The drawing under review shows one solid part. Ordinate dimensions are in mm from its lowest x, y, z. A direction names the side the tool comes from. Round coordinates to 2 decimals unless told otherwise and drop trailing zeros. Order: outer loops, then holes, each group sorted by start corner. A loop starts at its lowest first (then second) coordinate and runs counter-clockwise, first axis right, second up. Notation, with made-up numbers: (-8.75, 79) - (31.25, 79) arc R9 ccw to (31.25, 95) - close; hole circle Ø7 at (68, 47). An arc over 180 degrees is marked (long way). One line per question, with ' | ' between items.
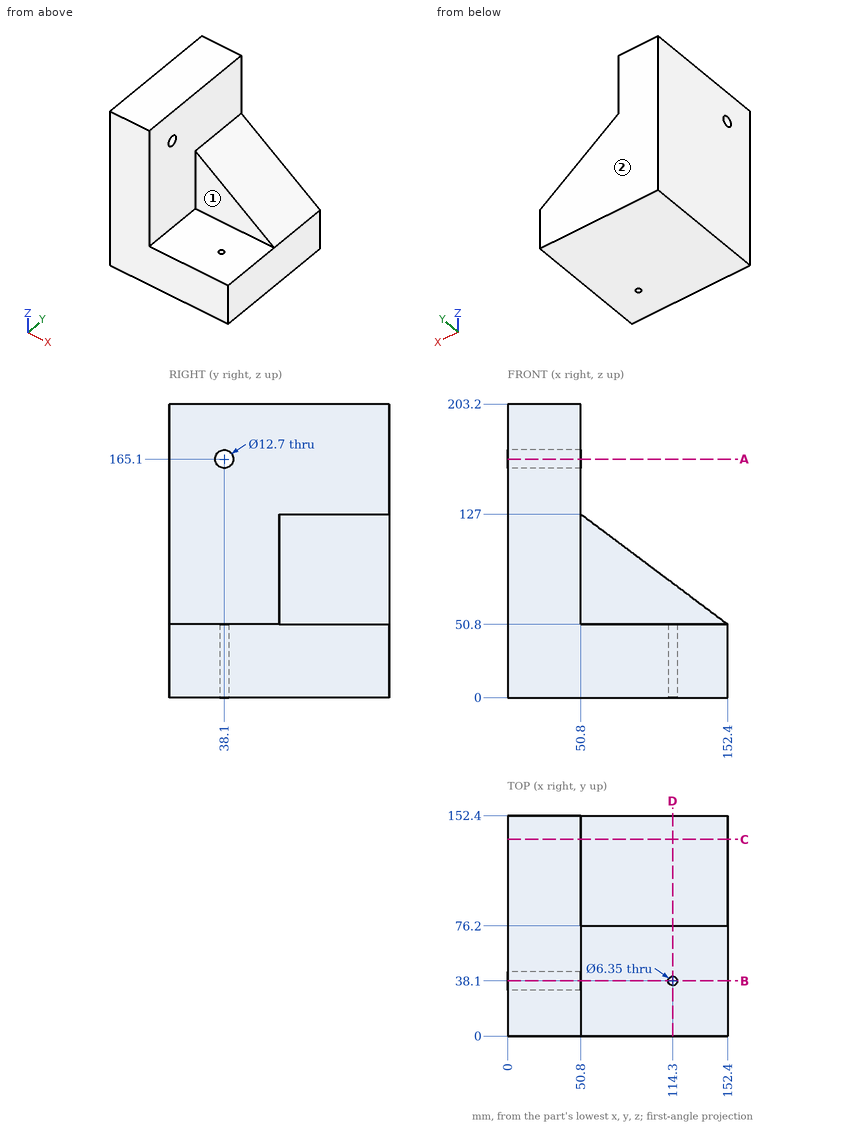
(1) We need section B-B on y = 38.1. State the section outline as (x, z) points (3 decimals), plus the area to 3 significant figures.
Output values:
outline: (0, 0) - (111.125, 0) - (111.125, 50.8) - (50.8, 50.8) - (50.8, 158.75) - (0, 158.75) - close; (0, 171.45) - (50.8, 171.45) - (50.8, 203.2) - (0, 203.2) - close; (117.475, 0) - (152.4, 0) - (152.4, 50.8) - (117.475, 50.8) - close | area: 14,500 mm^2
(2) For the marked faces 1 and 2, list the 3-axis set-ups (+Z, -Z, +X, -X, +Y, -Y) from which the entire face can be reached by the end or side of a thin tool; tool diameter is ignored.
Output values:
face 1: +Z, +X, -Y | face 2: +Z, -Z, +X, -X, +Y
(3) We need section D-D on x = 114.3. State the section outline as (y, z) points (3 decimals), plus the area to 3 significant figures.
Output values:
outline: (0, 0) - (34.925, 0) - (34.925, 50.8) - (0, 50.8) - close; (41.275, 0) - (152.4, 0) - (152.4, 79.375) - (76.2, 79.375) - (76.2, 50.8) - (41.275, 50.8) - close | area: 9,600 mm^2
(4) Insertion check: pin 1 (10 mm diameter, centred on x = 133, y = 99, fed in from +Z); pin 2 (23 mm diameter, centred on x = 124.5, y = 46, fed in from +Z); pin 3 (12 mm diameter, centred on x = 131, y = 106.5, fed in from +Z); pin 4 (6 mm diameter, centred on y = 100.5, z = 52, fed in from +X). Each pin has a flat end and moves straight along its axis. Give the tip position at first contact, or say it passes through.
Output values:
pin 1: z = 69.1 | pin 2: z = 50.8 | pin 3: z = 71.35 | pin 4: x = 152.4
(5) We need section C-C on y = 136. State the section outline as (x, z) points, plus the area to 3 significant figures.
Output values:
outline: (0, 0) - (152.4, 0) - (152.4, 50.8) - (50.8, 127) - (50.8, 203.2) - (0, 203.2) - close | area: 19,400 mm^2
(6) We need section A-A on z = 165.1. State the section outline as (x, y) points, plus the area to 3 significant figures.
Output values:
outline: (0, 0) - (50.8, 0) - (50.8, 31.75) - (0, 31.75) - close; (0, 44.45) - (50.8, 44.45) - (50.8, 152.4) - (0, 152.4) - close | area: 7,100 mm^2
(7) For probe 1 along Z at (x, y) = (33, 38); probe 2 along X at (y, z) = (38, 15); probe 3 along Y at (x, z) = (114, 18), list the stretches that pass through material, from the lowest coordinate up. Write a range as [from, to].
Output values:
probe 1: [0, 158.75], [171.45, 203.2] | probe 2: [0, 111.13], [117.47, 152.4] | probe 3: [0, 34.94], [41.26, 152.4]
